```python
from build123d import *

# Parameters (mm, degrees)
F0_W        = 127
F0_H        = 139.7
F1_DEPTH    = 107.95
F2_T1_DEPTH = 726.8985851792
F3_W        = 127
F3_H        = 63.5
F4_DEPTH    = 25.4
F5_W        = 76.2
F5_H        = 63.5
F6_DEPTH    = 50.8
F8_D        = 25.4
F10_D       = 25.4


# Not quite as in the source:
# - a fillet or chamfer that OpenCascade refuses, or shapes differently, is made with other operations: its cross-section is extruded or revolved along the edge and cut away or added


with BuildPart() as f1:
    # F0 (on Top) → F1 (new body)
    with BuildSketch(Plane.XY):
        with Locations((-63.5, 4.4167287707)):
            Rectangle(F0_W, F0_H)
    extrude(amount=F1_DEPTH)

    # F2: fillet of radius 120.65 on 1 edges, made by hand

    # F2_s2 → F2_t1 (cut)
    with BuildSketch(Plane.YZ.offset(-426.9492925896)):
        with BuildLine():
            ThreePointArc((74.2667287707, 0), (34.9844946572, 76.9902377631), (-45.7129882651, 107.95))
            Line((-45.7129882651, 107.95), (74.2667287707, 107.95))
            Line((74.2667287707, 107.95), (74.2667287707, 0))
        make_face()
    extrude(amount=F2_T1_DEPTH, mode=Mode.SUBTRACT)

    # F3 (on face) → F4 (join)
    with BuildSketch(Plane.XZ.offset(65.4332712293)):
        with Locations((-63.5, 76.2)):
            Rectangle(F3_W, F3_H)
    extrude(amount=F4_DEPTH)

    # F5 (on face) → F6 (join)
    with BuildSketch(Plane.XZ.offset(90.8332712293)):
        with Locations((-38.1, 76.2)):
            Rectangle(F5_W, F5_H)
    extrude(amount=F6_DEPTH)

    # F8 (through all)
    with Locations(Plane.XZ.offset(141.6332712293)):
        with Locations((-38.1, 76.2)):
            Hole(F8_D / 2)

    # F10 (through all)
    with Locations(Plane.YZ):
        with Locations((10.7667287707, 44.45)):
            Hole(F10_D / 2)


solid = f1.part
```
Work out the finished part from the listing and answer in its coordinate system (mm). A direction names the side the tool comes from. Coordinates: 2 decimals unless noted, no trailing zeros. Loops run counter-clockwise (first coordinate to the right, second up) from the corner with the lowest first, then second, coordinate; pieces in that order, holes last. Notation, with made-up numbers: (-13.75, 1) - (26.25, 1) arc R36 cw to (26.25, 37) - close; hole circle Ø2 at (15, 24). An arc over 180 degrees is marked (long way). Use a Markdown table: item, result.
Item 1: Consider probe 1 along Z at (x, y) = (-46.5, 0); probe 2 along X at (y, z) = (-35, 76); probe 3 along Z at (x, y) = (-38.1, -14.5). Determine where each line is inside the solid, lowest interval first. Write a range as from..to.
Evaluation:
| item | result |
|---|---|
| probe 1 | z = 0..37.71, 51.19..66.67, 85.73..98.95 |
| probe 2 | x = -127..-50.8, -25.4..0 |
| probe 3 | z = 0..63.5, 88.9..103.84 |
Item 2: Find section A-A, the plane x = -38.1. Determine the outline of the cut face in (y, z).
Evaluation:
| item | result |
|---|---|
| outline | (-141.63, 44.45) - (-65.43, 44.45) - (-65.43, 0) - (74.27, 0) arc R120.65 ccw to (47.83, 63.5) - (-141.63, 63.5) - close; (-141.63, 88.9) - (19.36, 88.9) arc R120.65 ccw to (-45.71, 107.95) - (-141.63, 107.95) - close; hole circle Ø25.4 at (10.77, 44.45) |
Item 3: Find section C-C, the plane x = -64.5. Determine the outline of the cut face in (y, z), and give its area (3 significant figures).
Evaluation:
| item | result |
|---|---|
| outline | (-141.63, 44.45) - (-65.43, 44.45) - (-65.43, 0) - (74.27, 0) arc R120.65 ccw to (-45.71, 107.95) - (-141.63, 107.95) - close; hole circle Ø25.4 at (10.77, 44.45) |
| area | 16,400 mm2 |
Item 4: Find section B-B, the plane y = -113. Determine the outline of the cut face in (x, z).
Evaluation:
| item | result |
|---|---|
| outline | (-76.2, 44.45) - (0, 44.45) - (0, 107.95) - (-76.2, 107.95) - close; hole circle Ø25.4 at (-38.1, 76.2) |
Item 5: Find section D-D, the plane z = 93. Determine the outline of the cut face in (x, y), and give its area (3 significant figures).
Evaluation:
| item | result |
|---|---|
| outline | (-127, -90.83) - (-76.2, -90.83) - (-76.2, -141.63) - (0, -141.63) - (0, 12.46) - (-127, 12.46) - close |
| area | 17,000 mm2 |
Item 6: The mould has two halves that part along Z. Classify faces 1 (the flat face through (-64, -65.433, 22)), 2 (the flat face through (-50, -95, 44.45)), 3 (the cylindrical face through (-64.39, 13.52, 32.05)): +Z half, -Z half, draft (parallel to the pull), parting line (faces both ways), or undercut.
Evaluation:
| item | result |
|---|---|
| face 1 | draft |
| face 2 | -Z half |
| face 3 | undercut |
Item 7: For faces 4 (the cylindrical face through (-64.39, 35.9, 76.16)), 5 (the flat face through (-76.2, -116, 76)), determine the directions among +Z, -Z, +X, -X, +Y, -Y from which every point of the face is accessible in a straight line to the end or side of a thin tool.
Evaluation:
| item | result |
|---|---|
| face 4 | +Z, +X, -X, +Y |
| face 5 | +Z, -Z, -X, -Y |
Item 8: Given pin 1 Ø12 at (x, z) = (-104, 13) entering from -Y; pin 2 Ø15 at (y, z) = (-128, 72.5) entering from -X; pin 3 Ø6 at (x, y) = (-73.5, -17.5) entering from +Z, each flat-ended and moving along its own axis, determine where each tip first touches the part or whether it passes through.
Evaluation:
| item | result |
|---|---|
| pin 1 | stops at y = -65.43 |
| pin 2 | stops at x = -76.2 |
| pin 3 | stops at z = 105.29 |
